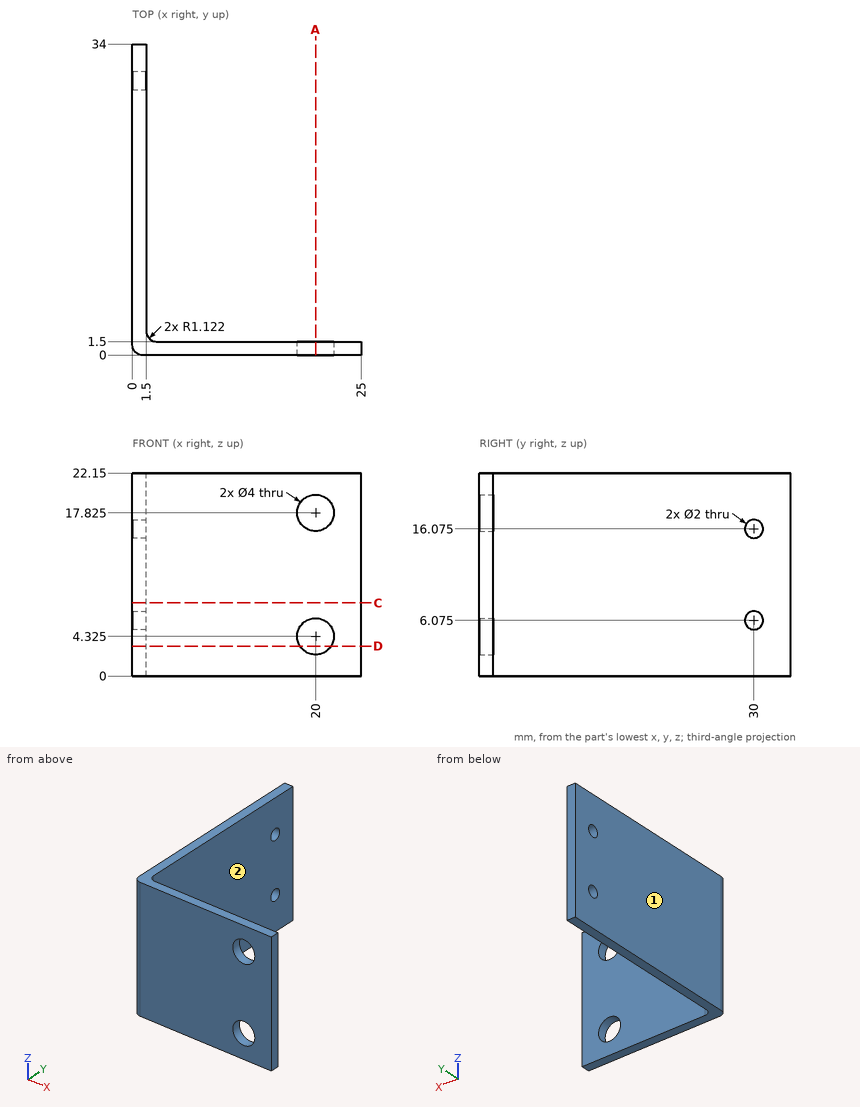
Verification items for this drawing (mm, ordinates from the low corner). A direction names the side the tool comes from. Give positions to 0.01 mm unless a question says otherwise; leave off trailing zeros. Order: outer loops, then holes, each group sorted by start corner. A loop starts at its lowest first (then second) coordinate and runs counter-clockwise, first axis right, second up. Notation, with made-up numbers: M -0.75,88.25 L 32.25,88.25 A22 cw 32.25,123.25 Z; hole C 43,5 d10. An arc over 180 degrees is marked long. Use a Markdown table: item, result.
Item 1: Material ranges on line 1 along Y through (x, z) = (5.25, 9); line 2 along Y through (x, z) = (1.75, 16) (1 decimal), recorded low to high.
Answers follow:
| item | result |
|---|---|
| line 1 | y = 0 to 1.5 |
| line 2 | y = 0 to 1.9 |
Item 2: Section check D-D (z = 3.25). Record the cut outline in (x, y) (1 decimal).
Answers follow:
| item | result |
|---|---|
| outline | M 0,1.1 A1.1 ccw 1.1,0 L 18.3,0 L 18.3,1.5 L 2.6,1.5 A1.1 cw 1.5,2.6 L 1.5,34 L 0,34 Z; M 21.7,0 L 25,0 L 25,1.5 L 21.7,1.5 Z |
Item 3: Section check C-C (z = 8). Record the cut outline in (x, y) (1 decimal).
Answers follow:
| item | result |
|---|---|
| outline | M 0,1.1 A1.1 ccw 1.1,0 L 25,0 L 25,1.5 L 2.6,1.5 A1.1 cw 1.5,2.6 L 1.5,34 L 0,34 Z |
Item 4: Tool access check on the marked faces 1 and 2. Record the directions out of +Z, -Z, +X, -X, +Y, -Y that give a thin tool (end or side, any length) a straight path to the whole face; none if there is none.
Answers follow:
| item | result |
|---|---|
| face 1 | +Z, -Z, -X, +Y, -Y |
| face 2 | +Z, -Z, +X, +Y |
Item 5: Section check A-A (x = 20). State how many separate pieces and enclosed holes the cut face has, and give its area (3 significant figures).
Answers follow:
| item | result |
|---|---|
| separate pieces | 3 |
| enclosed holes | 0 |
| area | 21.2 mm2 |
Item 6: Depth check by flat-ended pin: P1, Ø4, axis at y = 22.5, z = 3.5, coming from the -X side; P2, Ø2, axis at x = 6.5, z = 10.5, coming from the +Y side; P3, Ø2.5, axis at y = 30, z = 16.075, coming from the +X side. Enter the tip coordinate at first touch or a pass-through.
Answers follow:
| item | result |
|---|---|
| P1 | stops at x = 0 |
| P2 | stops at y = 1.5 |
| P3 | stops at x = 1.5 |
